CAD build for the part. Positions are in the model's coordinates, mm. Give positions to 0.01 mm unless a question says otherwise; leave off trailing zeros. Write each loop counter-clockwise with the first axis right and the second up, starting at its lowest first coordinate (ties: lowest second). Pieces come first, ordered by that corner, then holes. Notation, with made-up numbers: (12.5, 80) - (63.5, 80) arc R31 cw to (63.5, 119) - close; hole circle Ø5 at (44.25, 36.5). An arc over 180 degrees is marked (long way). Put each result on its own line as item: value. Start each with the question number.
1. Cut at D-D on y = -19.75. List the corners of the cut face in (x, z).
2. Cut at C-C on x = 13. List the corners of the cut face in (y, z).
3. Cut at B-B on x = -28. List the corners of the cut face in (y, z), and give its area (3 significant figures).
4. Drop flat-ended pins along their axis: pin 1 (2.5 mm diameter, centred on y = 15, z = 2.5, fed in from -X); pin 2 (1.9 mm diameter, centred on x = 28, y = -3.75, fed in from -Z); pin 3 (1.5 mm diameter, centred on y = 16.5, z = 1, fed in from +X); pin 4 (2 mm diameter, centred on x = -40.5, z = 2.5, fed in from +Y). Give the stop position or say it passes through.
5. Wall check: line 1 (Y direction, x = 28, z = 1.65); line 2 (Y direction, x = 9, z = 1.15); line 3 (Y direction, x = 15.5, z = 4.65). Give the ranges that are in metal, low to high.
6. Cut at A-A on y = -3.75. List the corners of the cut face in (x, z).
Autodesk Inventor part; units mm, degrees
ref_plane "YZ Plane" through (0, 0, 0) normal (1, 0, 0) x (0, 1, 0)
ref_plane "XZ Plane" through (0, 0, 0) normal (0, 1, 0) x (-1, 0, 0)
ref_plane "XY Plane" through (0, 0, 0) normal (0, 0, 1) x (1, 0, 0)
sketch "スケッチ1" plane through (0, 0, 0) normal (0, 0, 1) x (1, 0, 0)
  line L0 (-47, 28.25) -> (-37.7144, 28.25)
  line L1 (47, 28.25) -> (47, 23.75)
  line L2 (47, -28.25) -> (-47, -28.25)
  line L3 (-47, -28.25) -> (-47, -11.5167)
  line L4 (-47, 28.25) -> (47, -28.25) construction
  line L5 (47, 28.25) -> (-47, -28.25) construction
  line L6 (0, 28.25) -> (0, -28.25) construction
  line L7 (-52, 9.4167) -> (-52, -9.4167)
  line L8 (-52, 9.4167) -> (-47, 9.4167)
  arc A0 (-47, 9.4167) -> (-47, 11.5167) centre (-47, 10.4667) ccw
  line L9 (-47, 11.5167) -> (-47, 23.75)
  line L10 (-47, -11.5167) -> (-47, 11.5167)
  line L11 (52, 9.4167) -> (52, -9.4167)
  line L12 (52, 9.4167) -> (47, 9.4167)
  arc A1 (47, 11.5167) -> (47, 9.4167) centre (47, 10.4667) ccw
  line L13 (47, 11.5167) -> (47, -11.5167)
  line L14 (47, -11.5167) -> (47, -28.25)
  line L15 (-52, 0) -> (52, 0) construction
  line L16 (-52, -9.4167) -> (-47, -9.4167)
  arc A2 (-47, -11.5167) -> (-47, -9.4167) centre (-47, -10.4667) ccw
  arc A3 (47, -9.4167) -> (47, -11.5167) centre (47, -10.4667) ccw
  line L17 (52, -9.4167) -> (47, -9.4167)
  arc A4 (-47, 24.0838) -> (-37.7144, 28.25) centre (-44.75, 31.5) ccw
  arc A5 (37.7144, 28.25) -> (47, 24.0838) centre (44.75, 31.5) ccw
  line L18 (-47, 24.0838) -> (-47, 28.25)
  line L19 (-37.7144, 28.25) -> (47, 28.25)
  arc A6 (-37.7144, 28.25) -> (-47, 24.0838) centre (-44.75, 31.5) ccw
  arc A7 (47, 24.0838) -> (37.7144, 28.25) centre (44.75, 31.5) ccw
  line L20 (-44.75, 23.75) -> (-47, 23.75)
  line L21 (44.75, 23.75) -> (47, 23.75)
  line L22 (-47, 23.75) -> (-47, 24.0838)
  line L23 (47, 23.75) -> (47, 11.5167)
  line L24 (-30, -1.75) -> (30, -1.75) construction
  line L25 (30, -1.75) -> (30, -21.75) construction
  line L26 (30, -21.75) -> (-30, -21.75) construction
  line L27 (-30, -21.75) -> (-30, -1.75) construction
  line L28 (-30, -1.75) -> (30, -21.75) construction
  line L29 (30, -1.75) -> (-30, -21.75) construction
  circle A8 centre (-28, -3.75) radius 1.05
  line L30 (30, -11.75) -> (-30, -11.75) construction
  circle A9 centre (-28, -19.75) radius 1.05
  circle A10 centre (28, -3.75) radius 1.05
  circle A11 centre (28, -19.75) radius 1.05
  line L31 (-30.05, -1.7) -> (30.05, -1.7)
  line L32 (30.05, -1.7) -> (30.05, -21.8)
  line L33 (30.05, -21.8) -> (-30.05, -21.8)
  line L34 (-30.05, -21.8) -> (-30.05, -1.7)
  line L35 (-30.05, -1.7) -> (30.05, -21.8) construction
  line L36 (30.05, -1.7) -> (-30.05, -21.8) construction
  line L37 (-26, -5.75) -> (26, -5.75)
  line L38 (26, -5.75) -> (26, -17.75)
  line L39 (26, -17.75) -> (-26, -17.75)
  line L40 (-26, -17.75) -> (-26, -5.75)
  line L41 (-26, -5.75) -> (26, -17.75) construction
  line L42 (26, -5.75) -> (-26, -17.75) construction
  point P0 (0, 0)
  point P1 (0, 0)
  point P2 (0, 0)
  point P3 (0, 0)
  point P4 (47, 9.4167)
  point P5 (47, 9.4167)
  point P6 (0, -11.75)
  dimension "d0" = 94
  dimension "d1" = 56.5
  dimension "d10" = 1.05
  dimension "d11" = 5
  dimension "d34" = 18.8333
  dimension "d40" = 31.5
  dimension "d41" = 89.5
  dimension "d42" = 15.5
  dimension "d43" = 52
  dimension "d69" = 60
  dimension "d70" = 20
  dimension "d71" = 2
  dimension "d72" = 2
  dimension "d73" = 2.1
  dimension "d74" = 30
  dimension "d75" = 0.05
  dimension "d76" = 0.05
  dimension "d80" = 4
  dimension "d81" = 4
extrude "押し出し1" add sketch "スケッチ1" along normal blind 5 contours L19 A5 L21 L23 A1 L13 A3 L14 L2 L3 A2 L10 A0 L9 L20 A4
extrude "押し出し2" add sketch "スケッチ1" along normal blind 2.5 contours L10 L16 L7 L8 | L12 L11 L17 L13
sketch "スケッチ2" plane through (47, 11.5167, 0) normal (1, 0, 0) x (0, 0, -1)
  line L0 (0, -23.0333) -> (-5, -23.0333)
  line L1 (-2.5, -23.0333) -> (-2.5, -39.7667)
  line L2 (0, -39.7667) -> (-5, -39.7667)
  line L3 (0, -2.1) -> (-2.5, -2.1)
  line L4 (0, -20.9333) -> (-2.5, -20.9333)
  point P0 (0, -11.5167)
  point P1 (-2.5, 7.9)
  dimension "d67" = 10
hole "穴1" at (47, 19.4167, 2.5) direction (-1, 0, 0) diameter 2.459 depth 10 tip angle 118
sketch "スケッチ3" plane through (-47, 11.5167, 0) normal (-1, 0, 0) x (0, 0, 1)
  circle A0 centre (2.5, 7.9) radius 1.2295
  circle A1 centre (2.5, -30.9333) radius 1.2295
  point P0 (0, -11.5167)
  point P1 (2.5, 7.9)
hole "穴2" at (-47, 19.4167, 2.5) direction (1, 0, 0) diameter 2.459 depth 10 tip angle 118
extrude "押し出し3" add sketch "スケッチ1" along normal blind 3 contours L31 L32 L33 L34
fillet "フィレット1" radius 1 8 edges at (-30.05, -1.7, 4) (-30.05, -21.8, 4) (30.05, -21.8, 4) (30.05, -1.7, 4) (-26, -5.75, 1.5) (-26, -17.75, 1.5) (26, -5.75, 1.5) (26, -17.75, 1.5)
equation "\"d10\" = d4"
properties part number "Cockpit_horizontal_frame_05" material "アセタール樹脂、黒"
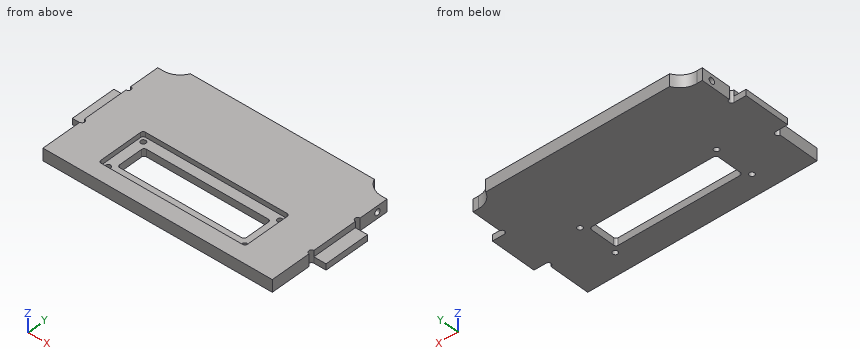
Report:
1. outline: (-47, 0) - (-29.05, 0) - (-29.05, 3) - (-30.05, 3) - (-30.05, 5) - (-47, 5) - close; (-26.95, 0) - (26.95, 0) - (26.95, 3) - (-26.95, 3) - close; (29.05, 0) - (47, 0) - (47, 5) - (30.05, 5) - (30.05, 3) - (29.05, 3) - close
2. outline: (-28.25, 0) - (-17.75, 0) - (-17.75, 3) - (-21.8, 3) - (-21.8, 5) - (-28.25, 5) - close; (-5.75, 0) - (28.25, 0) - (28.25, 5) - (-1.7, 5) - (-1.7, 3) - (-5.75, 3) - close
3. outline: (-28.25, 0) - (-20.8, 0) - (-20.8, 3) - (-21.8, 3) - (-21.8, 5) - (-28.25, 5) - close; (-18.7, 0) - (-4.8, 0) - (-4.8, 3) - (-18.7, 3) - close; (-2.7, 0) - (28.25, 0) - (28.25, 5) - (-1.7, 5) - (-1.7, 3) - (-2.7, 3) - close
3. area: 230 mm²
4. pin 1: stops at x = -47
4. pin 2: passes through
4. pin 3: stops at x = 47
4. pin 4: stops at y = 25.8
5. line 1: y = -28.25 to -20.8, -18.7 to -4.8, -2.7 to 28.25
5. line 2: y = -28.25 to -17.75, -5.75 to 28.25
5. line 3: y = -28.25 to -21.8, -1.7 to 28.25
6. outline: (-52, 0) - (-29.05, 0) - (-29.05, 3) - (-30.05, 3) - (-30.05, 5) - (-47, 5) - (-47, 2.5) - (-52, 2.5) - close; (-26.95, 0) - (26.95, 0) - (26.95, 3) - (-26.95, 3) - close; (29.05, 0) - (52, 0) - (52, 2.5) - (47, 2.5) - (47, 5) - (30.05, 5) - (30.05, 3) - (29.05, 3) - close
